```python
from build123d import *

# Parameters (mm, degrees)
BOSS_EXTRUDE1_DEPTH = 250
SHELL1_T            = -3
SKETCH4_R           = 4
CUT_EXTRUDE1_DEPTH  = 401
CUT_EXTRUDE3_DEPTH  = 400
CUT_EXTRUDE4_DEPTH  = 414
SKETCH7_W           = 291.024636147
SKETCH7_H           = 48.584181262
CUT_EXTRUDE5_DEPTH  = 232


with BuildPart() as part:
    # Sketch2 → Boss-Extrude1 (new body)
    with BuildSketch(Plane.XY):
        with BuildLine():
            Line((-140, -200), (150, -200))
            Line((150, -200), (150, 190))
            ThreePointArc((150, 190), (147.071067812, 197.071067812), (140, 200))
            Line((140, 200), (-140, 200))
            ThreePointArc((-140, 200), (-147.071067812, 197.071067812), (-150, 190))
            Line((-150, 190), (-150, -190))
            ThreePointArc((-150, -190), (-147.071067812, -197.071067812), (-140, -200))
        make_face()
    extrude(amount=BOSS_EXTRUDE1_DEPTH)

    # Shell1
    shell1_openings = [part.faces().sort_by_distance(p)[0] for p in [
        (-20.29586683, 27.438723973, 0),
    ]]
    offset(amount=SHELL1_T, openings=shell1_openings, kind=Kind.INTERSECTION)

    # Sketch4 → Cut-Extrude1 (cut, through all)
    with BuildSketch(Plane(origin=(0, 200, 0), x_dir=(1, 0, 0), z_dir=(0, 1, 0))):
        with Locations((-22.5, -130)):
            Circle(SKETCH4_R)
        with Locations((22.5, -130)):
            Circle(SKETCH4_R)
        with Locations((-22.5, -180)):
            Circle(SKETCH4_R)
        with Locations((22.5, -180)):
            Circle(SKETCH4_R)
    extrude(amount=-CUT_EXTRUDE1_DEPTH, mode=Mode.SUBTRACT)

    # Sketch6 → Cut-Extrude3 (cut)
    with BuildSketch(Plane(origin=(0, 200, 0), x_dir=(1, 0, 0), z_dir=(0, 1, 0))):
        with BuildLine():
            Line((-140, -39.142135624), (-140, 0))
            Line((-140, 0), (-150, 0))
            Line((-150, 0), (-150, -45))
            ThreePointArc((-150, -45), (-148.535533906, -41.464466094), (-145, -40))
            ThreePointArc((-145, -40), (-142.463470319, -39.783978395), (-140, -39.142135624))
        make_face()
    cut_extrude3 = extrude(amount=-CUT_EXTRUDE3_DEPTH, mode=Mode.SUBTRACT)

    # Sketch6<3> → Cut-Extrude4 (cut)
    with BuildSketch(Plane(origin=(0, 200, 0), x_dir=(1, 0, 0), z_dir=(0, 1, 0))):
        with BuildLine():
            Line((-130, -25), (-130, 0))
            Line((-130, 0), (-140, 0))
            Line((-140, 0), (-140, -39.142135624))
            ThreePointArc((-140, -39.142135624), (-132.752551286, -33.660254038), (-130, -25))
        make_face()
    cut_extrude4 = extrude(amount=-CUT_EXTRUDE4_DEPTH, mode=Mode.SUBTRACT)

    # Mirror1: Cut-Extrude3, Cut-Extrude4 across plane
    add(cut_extrude3.mirror(Plane(origin=(0, 0, 0), x_dir=(0, 0, 1), z_dir=(1, 0, 0))), mode=Mode.SUBTRACT)
    add(cut_extrude4.mirror(Plane(origin=(0, 0, 0), x_dir=(0, 0, 1), z_dir=(1, 0, 0))), mode=Mode.SUBTRACT)

    # Sketch7 → Cut-Extrude5 (cut)
    with BuildSketch(Plane(origin=(0, 200, 0), x_dir=(1, 0, 0), z_dir=(0, 1, 0))):
        with Locations((5.512318073, -14.850044993)):
            Rectangle(SKETCH7_W, SKETCH7_H)
    extrude(amount=-CUT_EXTRUDE5_DEPTH, mode=Mode.SUBTRACT)


solid = part.part
```
Design review of the part built by this model. Coordinates are the model's own, in mm. A direction names the side the tool comes from. Coordinates: 2 decimals unless noted, no trailing zeros. Write each loop counter-clockwise with the first axis right and the second up, starting at its lowest first coordinate (ties: lowest second). Pieces come first, ordered by that corner, then holes.
1) Add section A-A (z = 225). Write out the cut boundary in (x, y), plus the area to 3 significant figures.
2) Add section B-B (x = 73). Write out the cut boundary in (y, z), plus the area to 3 significant figures.
3) Machinability: for faces 4 (the flat face through (150, -8, 146)), 5 (the flat face through (1, -197, 122)), which of the approach directions +Z, -Z, +X, -X, +Y, -Y give a long, thin tool a straight path to every point of the face, cutting with its end or side? Answer none if there is none.
4) Mouldability with a two-part tool opening along Y and no side actions: class faces 1 (the flat face through (3, -200, 123)), 2 (the flat face through (2, 200, 143)), 3 (the flat face through (-147, 3, 142)) as +Y half, -Y half, draft (parallel to the pull), parting line (faces both ways), or undercut.
5) Insertion check: pin 1 (5 mm diameter, centred on x = -22.5, z = 130, fed in from +Y); pin 2 (0.9 mm diameter, centred on y = -199, z = 10.5, fed in from +X); pin 3 (3.5 mm diameter, centred on y = -199, z = 12.5, fed in from -X); pin 4 (1.5 mm diameter, centred on x = -44, y = -16.5, fed in from -Z). Each pin has a flat end and moves straight along its axis. Give the tip position at first contact, or say it passes through.
6) To check wall thickness, follow L1, parallel to Y at x = 13, z = 144; L2, parallel to Z at x = -22, y = 199; L3, parallel to X at y = 94, z = 101. State the ranges of each line that lie inside material, in increasing order.
7) Add section C-C (y = 35). Write out the cut boundary in (x, z).
Check result:
1. outline: (-150, -190) arc R10 ccw to (-140, -200) - (150, -200) - (150, 190) arc R10 ccw to (140, 200) - (-140, 200) arc R10 ccw to (-150, 190) - close; hole (-147, -190) arc R7 ccw to (-140, -197) - (147, -197) - (147, 190) arc R7 ccw to (140, 197) - (-140, 197) arc R7 ccw to (-147, 190) - close
1. area: 4,130 mm2
2. outline: (-200, 0) - (-197, 0) - (-197, 247) - (197, 247) - (197, 39.14) - (200, 39.14) - (200, 250) - (-200, 250) - close
2. area: 2,560 mm2
3. face 4: +Z, -Z, +X, +Y, -Y
3. face 5: -Z
4. face 1: -Y half
4. face 2: +Y half
4. face 3: undercut
5. pin 1: passes through
5. pin 2: stops at x = 130
5. pin 3: stops at x = -130
5. pin 4: stops at z = 247
6. L1: y = -200 to -197, 197 to 200
6. L2: z = 39.14 to 126.03, 133.97 to 176.03, 183.97 to 250
6. L3: x = -150 to -147, 147 to 150
7. outline: (-150, 45) arc R5 ccw to (-147, 40.42) - (-147, 247) - (147, 247) - (147, 40.42) arc R5 ccw to (150, 45) - (150, 250) - (-150, 250) - close
